```python
from build123d import *

# Parameters (mm, degrees)
BOSS_EXTRUDE2_DEPTH      = 25.4
BOSS_EXTRUDE2_DEPTH_BACK = 2.794
SKETCH1_W                = 101.6
SKETCH1_H                = 50.8
FILLET1_R                = 2.54


with BuildPart() as part:
    # Sketch1 → Boss-Extrude2 (new, two sides: drawn at the far end of the back side and taken through both)
    with BuildSketch(Plane(origin=(0, 0, 0), x_dir=(1, 0, 0), z_dir=(0, 1, 0)).offset(-BOSS_EXTRUDE2_DEPTH_BACK)):
        with BuildLine():
            ThreePointArc((56.621204677, 38.330630999), (82.021204677, 12.930630999), (56.621204677, -12.469369001))
            Line((56.621204677, -12.469369001), (56.621204677, 38.330630999))
        make_face()
        with Locations((5.821204677, 12.930630999)):
            Rectangle(SKETCH1_W, SKETCH1_H)
    extrude(amount=BOSS_EXTRUDE2_DEPTH + BOSS_EXTRUDE2_DEPTH_BACK)

    # Fillet1
    fillet1_edges = [part.edges().sort_by_distance(p)[0] for p in [
        (82.021204677, 25.4, -12.930630999),
        (5.821204677, 25.4, -38.330630999),
        (5.821204677, 25.4, 12.469369001),
    ]]
    fillet(fillet1_edges, radius=FILLET1_R)


solid = part.part
```
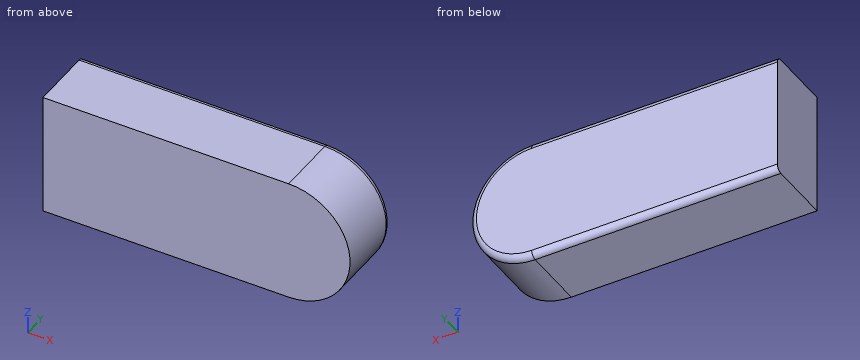
Can you work these out from the model? Positions are in its coordinate system, mm. Coordinates: 2 decimals unless noted, no trailing zeros. Order: outer loops, then holes, each group sorted by start corner. A loop starts at its lowest first (then second) coordinate and runs counter-clockwise, first axis right, second up.
1. I need wall thicknesses on line 1 (X direction, y = 21.5, z = -12); line 2 (Y direction, x = -7.5, z = 10.5); line 3 (X direction, y = -1, z = -21.5). Which ranges of each line are inside material? Lowest first, please.
2. I'm going to push flat-ended pins straight in: pin 1 (5 mm diameter, centred on y = 4, z = -4.5, fed in from +X); pin 2 (12 mm diameter, centred on y = 12.5, z = -20.5, fed in from +X). Where does each tip first touch, or does it pass through?
3. If we section it at A-A (y = 3.5): Please give me the cut outline in (x, z), then the cut area to 3 significant figures.
Entries:
1. line 1: x = -44.98 to 82
1. line 2: y = -2.79 to 25.34
1. line 3: x = -44.98 to 80.53
2. pin 1: stops at x = 81.32
2. pin 2: stops at x = 81.97
3. outline: (-44.98, -38.33) - (56.62, -38.33) arc R25.4 ccw to (56.62, 12.47) - (-44.98, 12.47) - close
3. area: 6,170 mm2
